Geometry check sheet. Reference: the model listing, model coordinates, mm. Face numbers are marked on the shaded views. A direction names the side the tool comes from. Round coordinates to 2 decimals unless told otherwise and drop trailing zeros. Loops run counter-clockwise (first coordinate to the right, second up) from the corner with the lowest first, then second, coordinate; pieces in that order, holes last. Notation, with made-up numbers: (35, 38.25) - (78, 38.25) arc R9 cw to (78, 46.25) - close; hole circle Ø1 at (48.5, 8). An arc over 180 degrees is marked (long way). Answer in a Markdown table with one row per item. Add a question column.
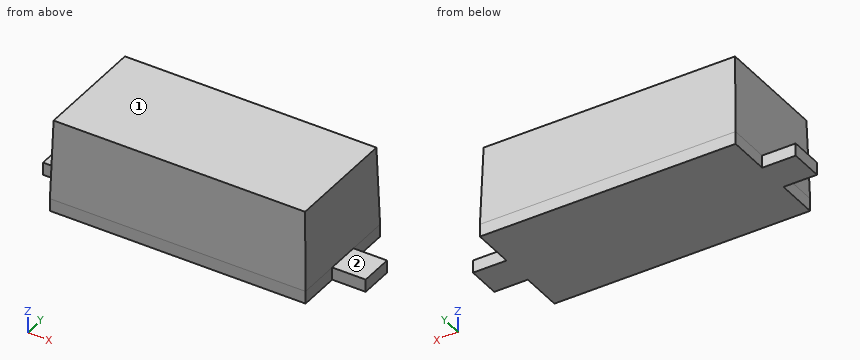
```python
from build123d import *

# Parameters (mm, degrees)
F1_DEPTH = 15
F3_DEPTH = 35
F4_W     = 8
F4_H     = 8
F5_DEPTH = 3


with BuildPart() as f1:
    # F0 (on Front) → F1 (new body, symmetric)
    with BuildSketch(Plane.XZ):
        Polygon((30, 22), (-30, 22), (-30.5, 3), (-30.5, 0), (30.5, 0), (30.5, 3), align=None)
    extrude(amount=F1_DEPTH, both=True)

    # F2 (on Right) → F3 (intersect, symmetric)
    with BuildSketch(Plane.YZ):
        Polygon((-14, 3), (-14, 0), (14, 0), (14, 3), (13.4, 22), (-13.4, 22), align=None)
    extrude(amount=F3_DEPTH, both=True, mode=Mode.INTERSECT)

    # F4 (on face) → F5 (join)
    with BuildSketch(Plane(origin=(0, 0, 0), x_dir=(1, 0, 0), z_dir=(0, 0, -1))):
        with Locations((34.5, 0)):
            Rectangle(F4_W, F4_H)
    extrude(amount=-F5_DEPTH)

    # F6: F1 across plane


with BuildPart() as f1_1:
    add(f1.part)
    add(f1.part.mirror(Plane.YZ))


solid = f1_1.part
```
Q1. Cross-section at A-A, the plane y = -0.25. Enter the section's corners in (x, z).
Q2. Scan lines: line 1 (X direction, y = -5, z = 1.5); line 2 (Z direction, x = -31, y = 2.25); line 3 (Y direction, x = 27.5, z = 8). Record each from-to range of solid material in increasing order. Write a range as from..to.
Q3. Cross-section at D-D, the plane y = 8. Enter the section's corners in (x, z).
Q4. Cross-section at B-B, the plane z = 1.5. Enter the section's corners in (x, y), plus the area to 3 significant figures.
Q5. Set-up check for the marked faces 1 and 2: record each of +Z, -Z, +X, -X, +Y, -Y from which the full face is reachable in a straight line by a thin tool's end or side.
Q6. Cross-section at C-C, the plane x = -14.5. Enter the section's corners in (y, z).
Q7. Depth check by flat-ended pin: P1, Ø8, axis at x = 29, z = 14.5, coming from the -Y side; P2, Ø6, axis at x = -20.5, y = -9.5, coming from the -Z side; P3, Ø1.5, axis at x = 26.5, z = 12, coming from the -Y side; P4, Ø12, axis at y = 9.5, z = 7, coming from the -X side. Enter the tip coordinate at first touch or a pass-through.
Check sheet entries:
| question | item | result |
|---|---|---|
| 1 | outline | (-38.5, 0) - (38.5, 0) - (38.5, 3) - (30.5, 3) - (30, 22) - (-30, 22) - (-30.5, 3) - (-38.5, 3) - close |
| 2 | line 1 | -30.5..30.5 |
| 2 | line 2 | 0..3 |
| 2 | line 3 | -13.84..13.84 |
| 3 | outline | (-30.5, 0) - (30.5, 0) - (30.5, 3) - (30, 22) - (-30, 22) - (-30.5, 3) - close |
| 4 | outline | (-38.5, -4) - (-30.5, -4) - (-30.5, -14) - (30.5, -14) - (30.5, -4) - (38.5, -4) - (38.5, 4) - (30.5, 4) - (30.5, 14) - (-30.5, 14) - (-30.5, 4) - (-38.5, 4) - close |
| 4 | area | 1,840 mm² |
| 5 | face 1 | +Z, +X, -X, +Y, -Y |
| 5 | face 2 | +Z, +X, +Y, -Y |
| 6 | outline | (-14, 0) - (14, 0) - (14, 3) - (13.4, 22) - (-13.4, 22) - (-14, 3) - close |
| 7 | P1 | y = -13.76 |
| 7 | P2 | z = 0 |
| 7 | P3 | y = -13.74 |
| 7 | P4 | x = -30.5 |
